Could you check a few things on this model? Use its own coordinates, in mm. A direction names the side the tool comes from. Coordinates: 2 decimals unless noted, no trailing zeros. Loops run counter-clockwise (first coordinate to the right, second up) from the corner with the lowest first, then second, coordinate; pieces in that order, holes last. Notation, with made-up numbers: (4, 12) -> (29, 12) arc R23 ccw to (29, 29) -> close; hole circle Ø6 at (-24.75, 74.25). An arc over 180 degrees is marked (long way). One line per question, with ' | ' between items. Start each with the question number.
(1) If we mould it in two halves opening along Z, with no side actions, what happens to faces 6 (the face through (-92.015, 2, 0)), 7 (the face through (92.015, 2, 0)), 8 (the face through (95.49, 6.54, -45.72)), 9 (the face through (-100, 6, 0))? For each: pulls with the +Z half, pulls with the -Z half, needs draft (parallel to the pull), parting line crosses it, or undercut.
(2) If I drill on line 1 along Z through (x, y) = (25.5, 1.5) (3 decimals); line 2 along X through (y, z) = (2.75, -5.5) (3 decimals); line 3 along Y through (x, z) = (44.5, -26), over which ranges is the centre line in solid material (lowest first)?
(3) Which directions (+Z, -Z, +X, -X, +Y, -Y) give clear straight access to the entire face, cutting with the end or side of a thin tool? Please do faces 1 (the face through (-1, 2, -45.015)), 2 (the face through (-90.5, 2.03, -40.74)), 3 (the face through (-87.5, 2.03, 37.74)), 4 (the face through (90.74, 2.03, -40.5)), 5 (the face through (-90.5, 2.03, 40.74)).
(4) Suppose I cut it at A-A (z = 13). Please give me the cut outline in (x, y) (3 decimals), plus the area to 3 significant figures.
(5) I'm going to push flat-ended pins straight in: pin 1 Ø1.2 at (x, y) = (3.5, 2.5) entering from +Z (3 decimals); pin 2 Ø2 at (x, y) = (-24.5, 1.5) entering from -Z (3 decimals); pin 3 Ø6 at (x, z) = (-13, -35.5) entering from -Y; pin 4 Ø4.5 at (y, z) = (2, 3) entering from +X. Where does each tip first touch, or does it pass through?
(6) Suppose I cut it at C-C (x = 68). Please give me the cut outline in (y, z) (3 decimals).
(7) Suppose I cut it at B-B (y = 1.5). Please give me the cut outline in (x, z) (3 decimals).
```python
from build123d import *

# Parameters (mm, degrees)
SKETCH1_W           = 190.03
SKETCH1_H           = 90.03
SKETCH1_W_2         = 184.03
SKETCH1_H_2         = 84.03
BOSS_EXTRUDE1_DEPTH = 4
SKETCH2_W           = 200
SKETCH2_H           = 100
BOSS_EXTRUDE2_DEPTH = 5
FILLET1_R           = 15


with BuildPart() as part:
    # Sketch1 → Boss-Extrude1 (new body)
    with BuildSketch(Plane(origin=(0, 0, 0), x_dir=(1, 0, 0), z_dir=(0, 1, 0))):
        Rectangle(SKETCH1_W, SKETCH1_H)
        Rectangle(SKETCH1_W_2, SKETCH1_H_2, mode=Mode.SUBTRACT)
    extrude(amount=BOSS_EXTRUDE1_DEPTH)

    # Sketch2 → Boss-Extrude2 (add)
    with BuildSketch(Plane(origin=(0, 4, 0), x_dir=(1, 0, 0), z_dir=(0, 1, 0))):
        Rectangle(SKETCH2_W, SKETCH2_H)
    extrude(amount=BOSS_EXTRUDE2_DEPTH)

    # Fillet1
    fillet1_edges = [part.edges().sort_by_distance(p)[0] for p in [
        (92.015, 2, 42.015),
        (92.015, 2, -42.015),
        (-92.015, 2, -42.015),
        (-92.015, 2, 42.015),
        (100, 6.5, 50),
        (100, 6.5, -50),
        (-100, 6.5, -50),
        (-100, 6.5, 50),
        (95.015, 2, 45.015),
        (-95.015, 2, 45.015),
        (-95.015, 2, -45.015),
        (95.015, 2, -45.015),
    ]]
    fillet(fillet1_edges, radius=FILLET1_R)


solid = part.part
```
Checks:
1) face 6: undercut | face 7: undercut | face 8: pulls with the -Z half | face 9: needs draft
2) line 1: z = -45.015 to -42.015, 42.015 to 45.015 | line 2: x = -95.015 to -92.015, 92.015 to 95.015 | line 3: y = 4 to 9
3) face 1: -Z, +X, -X, -Y | face 2: -Z, -X, -Y | face 3: -Y | face 4: -Z, +X, -Y | face 5: +Z, -X, -Y
4) outline: (-100, 4) -> (-95.015, 4) -> (-95.015, 0) -> (-92.015, 0) -> (-92.015, 4) -> (92.015, 4) -> (92.015, 0) -> (95.015, 0) -> (95.015, 4) -> (100, 4) -> (100, 9) -> (-100, 9) -> close | area: 1,020 mm^2
5) pin 1: stops at z = 45.015 | pin 2: stops at z = -45.015 | pin 3: stops at y = 4 | pin 4: stops at x = 100
6) outline: (0, -45.015) -> (4, -45.015) -> (4, -50) -> (9, -50) -> (9, 50) -> (4, 50) -> (4, 45.015) -> (0, 45.015) -> (0, 42.015) -> (4, 42.015) -> (4, -42.015) -> (0, -42.015) -> close
7) outline: (-95.015, -30.015) arc R15 ccw to (-80.015, -45.015) -> (80.015, -45.015) arc R15 ccw to (95.015, -30.015) -> (95.015, 30.015) arc R15 ccw to (80.015, 45.015) -> (-80.015, 45.015) arc R15 ccw to (-95.015, 30.015) -> close; hole (-92.015, -27.015) arc R15 ccw to (-77.015, -42.015) -> (77.015, -42.015) arc R15 ccw to (92.015, -27.015) -> (92.015, 27.015) arc R15 ccw to (77.015, 42.015) -> (-77.015, 42.015) arc R15 ccw to (-92.015, 27.015) -> close
